Build history of the part. All positions in model axes, mm. A direction names the side the tool comes from. Round coordinates to 2 decimals unless told otherwise and drop trailing zeros. Write each loop counter-clockwise with the first axis right and the second up, starting at its lowest first coordinate (ties: lowest second). Pieces come first, ordered by that corner, then holes. Notation, with made-up numbers: (51, 38.5) - (60, 38.5) arc R17 ccw to (60, 43.5) - close; hole circle Ø10 at (50.5, -8.5). An arc over 180 degrees is marked (long way). Answer as a JSON object with one key per item and string values. Group by question number.
Item 1: Two-plate mould, pull along X, no slides. Class faces 1 (the flat face through (-1, 6, 15)), 2 (the flat face through (-10.05, -10, 7)), 3 (the flat face through (-12.55, -8, 7)), 4 (the cylindrical face through (-10.415, -4.708, 7.395)): +X half, -X half, draft (parallel to the pull), parting line (faces both ways), or undercut.
Item 2: Which spindle directions (+Z, -Z, +X, -X, +Y, -Y) get a long thin tool onto all of the face, cutting with end or side? Do faces 5 (the flat face through (10.05, 2, 7)), 6 (the cylindrical face through (10.335, -14.249, 7.395)), 7 (the cylindrical face through (12.249, -14.265, 7.395)). Say none if no direction does.
Item 3: Flat gauge pins, fed straight in: pin 1 (0.8 mm diameter, centred on x = 8.5, z = 11, fed in from -Y); pin 2 (1.5 mm diameter, centred on x = 1, z = 10, fed in from -Y); pin 3 (2.5 mm diameter, centred on y = 3, z = 4.5, fed in from -X). Where does each tip first touch, or does it go through?
Item 4: Slice it at A-A, the plane y = -13. List the corners of the cut face in (x, z).
Item 5: Slice it at C-C, the plane x = -0.25. List the corners of the cut face in (y, z).
Item 6: Probe line 1 (X direction, y = -7.5, z = 11); line 2 (X direction, y = -3.75, z = 13); line 3 (X direction, y = 5.25, z = 6.5). List the from-to ranges inside material, lowest first. Write a range as from..to.
from build123d import *

# Parameters (mm, degrees)
SALIENTE_EXTRUIR1_DEPTH = 15
CROQUIS2_R              = 3
CORTAR_EXTRUIR1_DEPTH   = 20


with BuildPart() as part:
    # Croquis1 → Saliente-Extruir1 (new body)
    with BuildSketch(Plane.XY):
        with BuildLine():
            Line((-9.55, -5.05), (-8.05, -5.05))
            ThreePointArc((-8.05, -5.05), (-7.903553391, -4.696446609), (-7.55, -4.55))
            Line((-7.55, -4.55), (-7.55, 4.55))
            ThreePointArc((-7.55, 4.55), (-7.903553391, 5.403553391), (-7.05, 5.05))
            Line((-7.05, 5.05), (7.05, 5.05))
            ThreePointArc((7.05, 5.05), (7.903553391, 5.403553391), (7.55, 4.55))
            Line((7.55, 4.55), (7.55, -4.55))
            ThreePointArc((7.55, -4.55), (7.903553391, -4.696446609), (8.05, -5.05))
            Line((8.05, -5.05), (9.55, -5.05))
            ThreePointArc((9.55, -5.05), (10.403553391, -4.696446609), (10.05, -5.55))
            Line((10.05, -5.55), (10.05, -13.55))
            ThreePointArc((10.05, -13.55), (10.342893219, -14.257106781), (11.05, -14.55))
            Line((11.05, -14.55), (11.55, -14.55))
            ThreePointArc((11.55, -14.55), (12.257106781, -14.257106781), (12.55, -13.55))
            Line((12.55, -13.55), (12.55, -3.55))
            ThreePointArc((12.55, -3.55), (12.257106781, -2.842893219), (11.55, -2.55))
            Line((11.55, -2.55), (11.05, -2.55))
            ThreePointArc((11.05, -2.55), (10.342893219, -2.257106781), (10.05, -1.55))
            Line((10.05, -1.55), (10.05, 6.55))
            ThreePointArc((10.05, 6.55), (9.757106781, 7.257106781), (9.05, 7.55))
            Line((9.05, 7.55), (-9.05, 7.55))
            ThreePointArc((-9.05, 7.55), (-9.757106781, 7.257106781), (-10.05, 6.55))
            Line((-10.05, 6.55), (-10.05, -1.55))
            ThreePointArc((-10.05, -1.55), (-10.342893219, -2.257106781), (-11.05, -2.55))
            Line((-11.05, -2.55), (-11.55, -2.55))
            ThreePointArc((-11.55, -2.55), (-12.257106781, -2.842893219), (-12.55, -3.55))
            Line((-12.55, -3.55), (-12.55, -13.55))
            ThreePointArc((-12.55, -13.55), (-12.257106781, -14.257106781), (-11.55, -14.55))
            Line((-11.55, -14.55), (-11.05, -14.55))
            ThreePointArc((-11.05, -14.55), (-10.342893219, -14.257106781), (-10.05, -13.55))
            Line((-10.05, -13.55), (-10.05, -5.55))
            ThreePointArc((-10.05, -5.55), (-10.403553391, -4.696446609), (-9.55, -5.05))
        make_face()
    extrude(amount=SALIENTE_EXTRUIR1_DEPTH)

    # Croquis2 → Cortar-Extruir1 (cut)
    with BuildSketch(Plane(origin=(0, 7.55, 0), x_dir=(1, 0, 0), z_dir=(0, 1, 0))):
        with Locations(Location((0, -7.5, 0), (0, 0, 180))):
            Circle(CROQUIS2_R)
    extrude(amount=-CORTAR_EXTRUIR1_DEPTH, mode=Mode.SUBTRACT)


solid = part.part
Geometry says:
{
 "1": {"face 1": "draft", "face 2": "undercut", "face 3": "-X half", "face 4": "undercut"},
 "2": {"face 5": "+Z, -Z, +X, +Y", "face 6": "+Z, -Z, -Y", "face 7": "+Z, -Z, +X, -Y"},
 "3": {"pin 1": "stops at y = -5.05", "pin 2": "stops at y = 5.05", "pin 3": "stops at x = -10.05"},
 "4": {"outline": "(-12.55, 0) - (-10.05, 0) - (-10.05, 15) - (-12.55, 15) - close; (10.05, 0) - (12.55, 0) - (12.55, 15) - (10.05, 15) - close"},
 "5": {"outline": "(5.05, 0) - (7.55, 0) - (7.55, 4.51) - (5.05, 4.51) - close; (5.05, 10.49) - (7.55, 10.49) - (7.55, 15) - (5.05, 15) - close"},
 "6": {"line 1": "x = -12.55..-10.05, 10.05..12.55", "line 2": "x = -12.55..-7.55, 7.55..12.55", "line 3": "x = -10.05..-8.01, -7.09..-2.83, 2.83..7.09, 8.01..10.05"}
}
